from build123d import *

# Parameters (mm, degrees)
PAD_DEPTH       = 9
SKETCH001_R     = 8
PAD001_DEPTH    = 30
SKETCH002_R     = 6.5
POCKET_DEPTH    = 35
POCKET001_DEPTH = 5
CHAMFER_SIZE    = 1
FILLET_R        = 2
SKETCH004_W     = 5.296944
SKETCH004_H     = 3
POCKET002_DEPTH = 6
SKETCH005_R     = 1.65
HOLE_DEPTH      = 14.00858
HOLE_TIPS_R     = 1.65


with BuildPart() as part:
    # Sketch → Pad (new body)
    with BuildSketch(Plane.XY):
        with BuildLine():
            ThreePointArc((-5.656854, 5.656854), (0.011836, -7.999991), (5.64009, 5.673569))
            Line((5.64009, 14.673569), (5.64009, 5.673569))
            Line((-5.656854, 14.673569), (5.64009, 14.673569))
            Line((-5.656854, 5.656854), (-5.656854, 14.673569))
        make_face()
    extrude(amount=PAD_DEPTH)

    # Sketch001 (on Face5 of Pad) → Pad001 (join)
    with BuildSketch(Plane(origin=(0, 0, 0), x_dir=(1, 0, 0), z_dir=(0, 0, -1))):
        Circle(SKETCH001_R)
    extrude(amount=PAD001_DEPTH)

    # Sketch002 (on Face5 of Pad001) → Pocket (cut)
    with BuildSketch(Plane.XY.offset(9)):
        Circle(SKETCH002_R)
    extrude(amount=-POCKET_DEPTH, mode=Mode.SUBTRACT)

    # Sketch003 (on Face8 of Pocket) → Pocket001 (cut)
    with BuildSketch(Plane(origin=(0, 0, -30), x_dir=(1, 0, 0), z_dir=(0, 0, -1))):
        with BuildLine():
            Line((-1.930765, 1.588126), (1.930765, 1.588126))
            ThreePointArc((2.063156, -1.411874), (2.497569, 0.110218), (1.930765, 1.588126))
            Line((-2.063156, -1.411874), (2.063156, -1.411874))
            ThreePointArc((-1.930765, 1.588126), (-2.497569, 0.110218), (-2.063156, -1.411874))
        make_face()
    extrude(amount=-POCKET001_DEPTH, mode=Mode.SUBTRACT)

    # Chamfer
    chamfer_edges = [part.edges().sort_by_distance(p)[0] for p in [
        (-8, 0, -30),
    ]]
    chamfer(chamfer_edges, length=CHAMFER_SIZE)

    # Fillet
    fillet_edges = [part.edges().sort_by_distance(p)[0] for p in [
        (5.64009, 14.673569, 4.5),
        (-5.656854, 14.673569, 4.5),
    ]]
    fillet(fillet_edges, radius=FILLET_R)

    # Sketch004 (on Face9 of Fillet) → Pocket002 (cut)
    with BuildSketch(Plane.XY.offset(9)):
        with Locations((-0.008382, 10.173569)):
            Rectangle(SKETCH004_W, SKETCH004_H)
    extrude(amount=-POCKET002_DEPTH, mode=Mode.SUBTRACT)

    # Sketch005 (on Face5 of Pocket002) → Hole (cut)
    with BuildSketch(Plane(origin=(0, 14.673569, 0), x_dir=(-1, 0, 0), z_dir=(0, 1, 0))):
        with Locations((0, 6)):
            Circle(SKETCH005_R)
    extrude(amount=-HOLE_DEPTH, mode=Mode.SUBTRACT)

    # Hole tips → Hole tip 1 section 0
    with BuildSketch(Plane(origin=(0, 0.664989, 0), x_dir=(-1, 0, 0), z_dir=(0, 1, 0)), mode=Mode.PRIVATE) as hole_tip_1_s0:
        with Locations((0, 6)):
            Circle(HOLE_TIPS_R)
    loft([hole_tip_1_s0.sketch, Vertex(0, -0.326431, 6)], mode=Mode.SUBTRACT)


solid = part.part
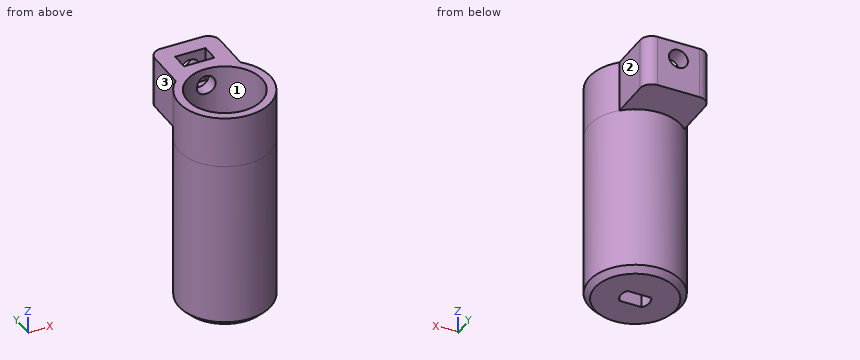
Geometry check sheet. Reference: the model listing, model coordinates, mm. Face numbers are marked on the shaded views. A direction names the side the tool comes from. Round coordinates to 2 decimals unless told otherwise and drop trailing zeros. Write each loop counter-clockwise with the first axis right and the second up, starting at its lowest first coordinate (ties: lowest second). Pieces come first, ordered by that corner, then holes.
Item 1: Section check B-B (x = 0). Record the boundary of the cut face in (y, z), plus the area to 3 significant figures.
Determined:
outline: (-8, -29) - (-7, -30) - (-1.59, -30) - (-1.59, -26) - (-6.5, -26) - (-6.5, 9) - (-8, 9) - close; (1.41, -30) - (7, -30) - (8, -29) - (8, 0) - (14.67, 0) - (14.67, 4.35) - (11.67, 4.35) - (11.67, 3) - (8.67, 3) - (8.67, 4.35) - (6.5, 4.35) - (6.5, -26) - (1.41, -26) - close; (6.5, 7.65) - (8.67, 7.65) - (8.67, 9) - (6.5, 9) - close; (11.67, 7.65) - (14.67, 7.65) - (14.67, 9) - (11.67, 9) - close
area: 181 mm2
Item 2: Section check D-D (y = 9.75). Record the boundary of the cut face in (x, z), plus the area to 3 significant figures.
Determined:
outline: (-5.66, 0) - (5.64, 0) - (5.64, 9) - (2.64, 9) - (2.64, 3) - (-2.66, 3) - (-2.66, 9) - (-5.66, 9) - close
area: 69.9 mm2
Item 3: Material ranges on line 1 along Z through (x, y) = (0, 13.7); line 2 along Z through (x, y) = (-3, 3.25); line 3 along Y through (x, z) = (3, -7.5), recorded low to high.
Determined:
line 1: z = 0 to 4.35, 7.65 to 9
line 2: z = -30 to -26
line 3: y = -7.42 to -5.77, 5.77 to 7.42
Item 4: Section check A-A (y = 0). Record the boundary of the cut face in (x, z), plus the area to 3 significant figures.
Determined:
outline: (-8, -29) - (-7, -30) - (-2.5, -30) - (-2.5, -26) - (-6.5, -26) - (-6.5, 9) - (-8, 9) - close; (2.5, -30) - (7, -30) - (8, -29) - (8, 9) - (6.5, 9) - (6.5, -26) - (2.5, -26) - close
area: 148 mm2
Item 5: Access from +Z, -Z, +X, -X, +Y, -Y to the whole of each face (thin tool, end or side, straight path). Record for the marked faces 1, 2 and 3.
Determined:
face 1: +Z
face 2: +Z, -Z, +X, +Y
face 3: +Z, -Z, -X, +Y
Item 6: Go/stop test with flat-tipped pins: pin 1 Ø4 at (x, y) = (2, -3) entering from +Z; pin 2 Ø2.5 at (x, y) = (-2.5, 8.5) entering from -Z; pin 3 Ø3.5 at (y, z) = (9.5, 4.5) entering from +X. Record where each tip stops, or that it passes through.
Determined:
pin 1: stops at z = -26
pin 2: stops at z = -29.39
pin 3: stops at x = 5.64
Item 7: Section check C-C (z = 6). Record the boundary of the cut face in (x, y), plus the area to 3 significant figures.
Determined:
outline: (-5.66, 5.66) arc R8 ccw (long way) to (5.64, 5.67) - (5.64, 12.67) arc R2 ccw to (3.64, 14.67) - (1.65, 14.67) - (1.65, 11.67) - (2.64, 11.67) - (2.64, 8.67) - (1.65, 8.67) - (1.65, 6.29) arc R6.5 cw (long way) to (-1.65, 6.29) - (-1.65, 8.67) - (-2.66, 8.67) - (-2.66, 11.67) - (-1.65, 11.67) - (-1.65, 14.67) - (-3.66, 14.67) arc R2 ccw to (-5.66, 12.67) - close
area: 117 mm2
